Source: CAD feature listing. Evaluate the final solid. Frame: model axes, mm. A direction names the side the tool comes from. Give positions to 0.01 mm unless a question says otherwise; leave off trailing zeros. Loops run counter-clockwise (first coordinate to the right, second up) from the corner with the lowest first, then second, coordinate; pieces in that order, holes last. Notation, with made-up numbers: M 81,-9 L 136,-9 A21 cw 136,27 Z; hole C 47.5,25.25 d7. An arc over 180 degrees is marked long. Answer in a Markdown table with one row per item.
Autodesk Inventor part; units mm, degrees
ref_plane "YZ Plane" through (0, 0, 0) normal (1, 0, 0) x (0, 1, 0)
ref_plane "XZ Plane" through (0, 0, 0) normal (0, 1, 0) x (-1, 0, 0)
ref_plane "XY Plane" through (0, 0, 0) normal (0, 0, 1) x (1, 0, 0)
sketch "スケッチ1" plane through (0, 0, 0) normal (0, 1, 0) x (-1, 0, 0)
  line L0 (-35.3553, 0) -> (0, 35.3553)
  line L1 (0, 35.3553) -> (35.3553, 0)
  line L2 (35.3553, 0) -> (0, -35.3553)
  line L3 (0, -35.3553) -> (-35.3553, 0)
  line L4 (-25, 25) -> (25, -25) construction
  line L5 (25, 25) -> (-25, -25) construction
  line L6 (0, 0) -> (0, -30)
  line L7 (0, -30) -> (5.3553, -30)
  line L8 (5.3553, -30) -> (10.7107, -35.3553)
  line L9 (5.3553, -30) -> (5.3553, 0)
  line L10 (0, 0) -> (30, 0)
  line L11 (30, 0) -> (30, -5.3553)
  line L12 (30, -5.3553) -> (0, -5.3553)
  line L13 (35.3553, 0) -> (47.1243, -11.769)
  line L14 (35.3553, 0) -> (35.3553, -35.3553)
  line L15 (0, -35.3553) -> (35.3553, -35.3553)
  line L16 (30, -5.3553) -> (35.3553, -10.7107)
  line L17 (5.3553, 30) -> (5.3553, 0)
  line L18 (30, 5.3553) -> (0, 5.3553)
  line L19 (0, 35.3553) -> (35.3553, 0)
  line L20 (30, 5.3553) -> (35.3553, 10.7107)
  line L21 (30, 0) -> (30, 5.3553)
  line L22 (0, 30) -> (5.3553, 30)
  line L23 (5.3553, 30) -> (10.7107, 35.3553)
  line L24 (0, 35.3553) -> (35.3553, 35.3553)
  line L25 (35.3553, 0) -> (35.3553, 35.3553)
  line L26 (0, 0) -> (0, 30)
  line L27 (0, 0) -> (30, 0)
  line L28 (-30, 5.3553) -> (0, 5.3553)
  line L29 (-5.3553, 30) -> (-5.3553, 0)
  line L30 (-35.3553, 0) -> (0, 35.3553)
  line L31 (-5.3553, 30) -> (-10.7107, 35.3553)
  line L32 (0, 30) -> (-5.3553, 30)
  line L33 (-30, 0) -> (-30, 5.3553)
  line L34 (-30, 5.3553) -> (-35.3553, 10.7107)
  line L35 (-35.3553, 0) -> (-35.3553, 35.3553)
  line L36 (0, 35.3553) -> (-35.3553, 35.3553)
  line L37 (0, 0) -> (-30, 0)
  line L38 (0, 0) -> (0, 30)
  line L39 (-5.3553, -30) -> (-5.3553, 0)
  line L40 (-30, -5.3553) -> (0, -5.3553)
  line L41 (0, -35.3553) -> (-35.3553, 0)
  line L42 (-30, -5.3553) -> (-35.3553, -10.7107)
  line L43 (-30, 0) -> (-30, -5.3553)
  line L44 (0, -30) -> (-5.3553, -30)
  line L45 (-5.3553, -30) -> (-10.7107, -35.3553)
  line L46 (0, -35.3553) -> (-35.3553, -35.3553)
  line L47 (-35.3553, 0) -> (-35.3553, -35.3553)
  line L48 (0, 0) -> (0, -30)
  line L49 (0, 0) -> (-30, 0)
  point P0 (35.3553, 0)
  point P1 (5.3553, 5.3553)
  point P2 (-5.3553, 5.3553)
  point P3 (-5.3553, -5.3553)
  point P4 (0, -35.3553)
  point P5 (5.3553, -5.3553)
  dimension "d0" = 50
  dimension "d1" = 50
  dimension "d3" = 30
  dimension "d4" = 30
  dimension "d7" = 360
extrude "押し出し1" add sketch "スケッチ1" along normal mid plane 8 contours L35 L34 L0 | L0 L33 L43 L3 | L3 L42 L47 | L28 L29 L37 L33 | L43 L37 L39 L40 | L31 L36 L0 | L32 L26 L28 L29 | L0 L1 L22 L32 | L28 L26 L37 L29 | L44 L7 L2 L3 | L39 L40 L6 L44 | L3 L46 L45 | L39 L37 L6 L40 | L24 L23 L1 | L22 L17 L18 L26 | L18 L17 L10 L26 | L2 L8 L15 | L6 L12 L9 L7 | L6 L10 L9 L12 | L18 L21 L10 L17 | L9 L10 L11 L12 | L20 L25 L1 | L1 L2 L11 L21 | L2 L14 L16
sketch "スケッチ3" plane through (5.3553, -4, 30) normal (0.7071, 0, -0.7071) x (-0.7071, 0, -0.7071)
  line L0 (-7.5736, 8) -> (7.5736, 8)
  line L1 (17.4264, 0) -> (0, 0)
  line L2 (-7.5736, 8) -> (0, 0)
  line L3 (-7.5736, 0) -> (7.5736, 0)
  line L4 (0, 8) -> (-7.5736, 0)
  circle A0 centre (-3.7868, 4) radius 3
  point P0 (25, 4)
  dimension "d12" = 6
extrude "押し出し2" add sketch "スケッチ3" along normal blind 35 contours A0 L4 L2 | L2 L4 A0 | A0 L2 L4 | L2 A0 L4
pattern_circular "円形状パターン1" count 4 over 360 about axis through (0, -10, 0) along (0, 1, 0) of "押し出し2"
sketch "スケッチ4" plane through (0, 4, 0) normal (0, 1, 0) x (1, 0, 0)
  line L0 (-30, -5.3553) -> (-5.3553, -5.3553)
  line L1 (-35.3553, -10.7107) -> (-30, -5.3553)
  arc A0 (-5.3553, -5.3553) -> (-30, -5.3553) centre (-17.6777, -37.7141) ccw
  line L2 (-30, -5.3553) -> (-5.3553, -5.3553)
  line L3 (-35.3553, 0) -> (35.3553, 0)
  line L4 (35.3553, -10.7107) -> (35.3553, 10.7107)
  line L5 (10.7107, 35.3553) -> (-10.7107, 35.3553)
  line L6 (0, 35.3553) -> (0, -35.3553)
  arc A1 (-30, 5.3553) -> (-5.3553, 5.3553) centre (-17.6777, 37.7141) ccw
  arc A2 (5.3553, -5.3553) -> (5.3553, -30) centre (37.7141, -17.6777) ccw
  line L7 (5.3553, -30) -> (5.3553, -5.3553)
  arc A3 (-5.3553, -30) -> (-5.3553, -5.3553) centre (-37.7141, -17.6777) ccw
  arc A4 (5.3553, 5.3553) -> (30, 5.3553) centre (17.6777, 37.7141) ccw
  line L8 (30, 5.3553) -> (5.3553, 5.3553)
  arc A5 (30, -5.3553) -> (5.3553, -5.3553) centre (17.6777, -37.7141) ccw
  arc A6 (-5.3553, 5.3553) -> (-5.3553, 30) centre (-37.7141, 17.6777) ccw
  line L9 (-5.3553, 30) -> (-5.3553, 5.3553)
  arc A7 (5.3553, 30) -> (5.3553, 5.3553) centre (37.7141, 17.6777) ccw
  line L10 (-30, 5.3553) -> (-35.3553, 10.7107)
  line L11 (-30, 5.3553) -> (-5.3553, 5.3553)
  line L12 (-30, 5.3553) -> (-5.3553, 5.3553)
  line L13 (-5.3553, 30) -> (-5.3553, 5.3553)
  line L14 (5.3553, 30) -> (5.3553, 5.3553)
  line L15 (5.3553, -5.3553) -> (30, -5.3553)
  line L16 (10.7107, -35.3553) -> (5.3553, -30)
  line L17 (5.3553, -5.3553) -> (5.3553, -30)
  line L18 (-5.3553, -5.3553) -> (-5.3553, -30)
  point P0 (0, 0)
  point P1 (-5.3553, 5.3553)
  point P2 (-5.3553, 5.3553)
  point P3 (5.3553, 5.3553)
  point P4 (5.3553, 5.3553)
  point P5 (5.3553, 5.3553)
  point P6 (5.3553, 5.3553)
  dimension "d20" = 360
extrude "押し出し3" cut sketch "スケッチ4" against normal blind 8
sketch "スケッチ5" plane through (0, 4, 0) normal (0, 1, 0) x (1, 0, 0)
  circle A0 centre (0, 0) radius 15
  circle A1 centre (0, 0) radius 12
  circle A2 centre (0, 0) radius 8
  circle A3 centre (0, 0) radius 3
  dimension "d24" = 30
  dimension "d25" = 6
  dimension "d26" = 24
  dimension "d27" = 16
extrude "押し出し4" add sketch "スケッチ5" against normal blind 8 contours A0 | A2 | A3
sketch "スケッチ6" plane through (0, 4, 0) normal (0, 1, 0) x (1, 0, 0)
  circle A0 centre (0, 0) radius 3
  dimension "d30" = 6
extrude "押し出し5" cut sketch "スケッチ6" against normal blind 8
Q1. Contact query for flat-ended pins moving along their axis: pin 1 Ø6 at (x, z) = (-8.5, -24.5) entering from +Y; pin 2 Ø12 at (x, z) = (-20, -17) entering from +Y; pin 3 Ø3 at (x, z) = (1, 0.5) entering from -Y; pin 4 Ø1.5 at (x, z) = (27.5, 16.5) entering from +Y. Output: stop coordinate, or through.
Values follow:
| item | result |
|---|---|
| pin 1 | y = 1.73 |
| pin 2 | y = 3 |
| pin 3 | through |
| pin 4 | y = 2.55 |
Q2. Section query C-C (x = -8). Give the number of separate pieces and of enclosed holes in the cut face, plus the area to 3 significant figures.
Values follow:
| item | result |
|---|---|
| separate pieces | 5 |
| enclosed holes | 0 |
| area | 214 mm^2 |
Q3. Section query B-B (x = 0). Output: boundary loops of the cut face in (y, z).
Values follow:
| item | result |
|---|---|
| outline | M -4,-35.36 L 4,-35.36 L 4,-3 L -4,-3 Z; M -4,3 L 4,3 L 4,35.36 L -4,35.36 Z |
Q4. Ray query, probe 1 along X at (y, z) = (1.5, 0); probe 2 along Z at (x, y) = (-26, -2). Return the intervals inside material, ascending. Write a range as from..to.
Values follow:
| item | result |
|---|---|
| probe 1 | -35.36..-3, 3..35.36 |
| probe 2 | -17.87..-11.55, -4.1..4.1, 11.55..17.87 |
Q5. Mould query, pull axis X, two halves, no side actions, for faces 4 (the cylindrical face through (-8.83, 0.06, -4.24)), 5 (the flat face through (0, 0, 35.355)), 6 (the flat face through (-35.355, 0, 0)). Classes: +X half, -X half, draft (parallel to the pull), parting line (faces both ways), or undercut.
Values follow:
| item | result |
|---|---|
| face 4 | undercut |
| face 5 | draft |
| face 6 | -X half |
Q6. Section query A-A (z = 0). Output: boundary loops of the cut face in (x, y).
Values follow:
| item | result |
|---|---|
| outline | M -35.36,-4 L -3,-4 L -3,4 L -35.36,4 Z; M 3,-4 L 35.36,-4 L 35.36,4 L 3,4 Z |
Q7. Reachability of faces 1 (the flat face through (0, 0, -35.355)), 2 (the cylindrical face through (22.554, 0.056, 3.434)), 3 (the flat face through (30.855, -1.834, 6.21)) from +Z, -Z, +X, -X, +Y, -Y: full face, straight path, thin tool, end or side. Return the list, or none.
Values follow:
| item | result |
|---|---|
| face 1 | -Z, +X, -X, +Y, -Y |
| face 2 | +Y, -Y |
| face 3 | none |
